```python
from build123d import *

# Parameters (mm, degrees)
SKETCH1_W                                      = 152.4
SKETCH1_H                                      = 152.4
BOSS_EXTRUDE1_DEPTH                            = 12.7
F_2_56_TAPPED_HOLE1_D                          = 1.778
CBORE_FOR_4_SOCKET_HEAD_CAP_SCREW1_D           = 3.2639
CBORE_FOR_4_SOCKET_HEAD_CAP_SCREW1_CBORE_D     = 5.55752
CBORE_FOR_4_SOCKET_HEAD_CAP_SCREW1_CBORE_DEPTH = 2.8448
F_6_0MM_DOWEL_HOLE1_D                          = 6
F_8_0MM_DOWEL_HOLE1_D                          = 8
F_1_4_20_TAPPED_HOLE1_D                        = 5.1054


with BuildPart() as part:
    # Sketch1 → Boss-Extrude1 (new body)
    with BuildSketch(Plane.XY):
        Rectangle(SKETCH1_W, SKETCH1_H)
    extrude(amount=BOSS_EXTRUDE1_DEPTH)

    # #2-56 Tapped Hole1 (through all)
    with Locations(Plane.XY.offset(12.7)):
        with Locations((-50.8, 0), (-50.8, -58), (-1.8, -58), (-1.8, 0)):
            Hole(F_2_56_TAPPED_HOLE1_D / 2)

    # CBORE for #4 Socket Head Cap Screw1 (through all)
    with Locations(Plane.XY.offset(12.7)):
        with Locations((-73.025, 63.5), (-73.025, 73.025), (73.025, 63.5), (73.025, 73.025), (73.025, -63.5), (73.025, -73.025), (-73.025, -63.5), (-73.025, -73.025)):
            CounterBoreHole(CBORE_FOR_4_SOCKET_HEAD_CAP_SCREW1_D / 2, CBORE_FOR_4_SOCKET_HEAD_CAP_SCREW1_CBORE_D / 2, CBORE_FOR_4_SOCKET_HEAD_CAP_SCREW1_CBORE_DEPTH)

    # Ø6.0mm Dowel Hole1 (through all)
    with Locations(Plane.XY.offset(12.7)):
        with Locations((57.15, 63.5), (57.15, -24.801), (-19.32090918, 19.3495), (57.15, -57.15), (25.4, -57.15)):
            Hole(F_6_0MM_DOWEL_HOLE1_D / 2)

    # Ø8.0mm Dowel Hole1 (through all)
    with Locations(Plane.XY.offset(12.7)):
        with Locations((31.65969694, 19.3495)):
            Hole(F_8_0MM_DOWEL_HOLE1_D / 2)

    # 1/4-20 Tapped Hole1 (through all)
    with Locations(Plane.XY.offset(12.7)):
        with Locations((31.65969694, 0.2995), (31.65969694, 38.3995)):
            Hole(F_1_4_20_TAPPED_HOLE1_D / 2)


solid = part.part
```
CAD build for the part. Positions are in the model's coordinates, mm. A direction names the side the tool comes from. Give positions to 0.01 mm unless a question says otherwise; leave off trailing zeros. Order: outer loops, then holes, each group sorted by start corner. A loop starts at its lowest first (then second) coordinate and runs counter-clockwise, first axis right, second up.
(1) Saw through at A-A, the plane x = 57.15. Give the cut face in (y, z).
(2) Tool access for faces 1 (the cylindrical face through (-75.8, 73.15, 11.3)), 2 (the cylindrical face through (27.844, 20.551, 6.261)): list every direction of +Z, -Z, +X, -X, +Y, -Y with a clear straight run to the whole face (end or side of a thin tool).
(3) Flat gauge pins, fed straight in: pin 1 (4.5 mm diameter, centred on x = 73.5, y = 64.5, fed in from +Z); pin 2 (5 mm diameter, centred on x = 73.025, y = -73.025, fed in from +Z). Where does each tip first touch, or does it go through?
(4) Saw through at B-B, the plane x = -19. Give the cut face in (y, z), then the cut area to 3 significant figures.
(5) Drill centre lines: L1, parallel to X at y = 37.5, z = 2.5; L2, parallel to X at y = 23, z = 10.25. Where is each one in solid material? Low to high.
(6) Mould opens along X. For faces 3 (the flat face through (-1, -76.2, 6)), 4 (the cylindrical face through (-16.324, 19.481, 6.261)), 5 (the flat face through (76.2, -1, 6)), 6 (the cylindrical face through (73.237, -71.407, 4.859)) say: released by +X, released by -X, zero draft, split by the parting line, or undercut.
Results found:
1. outline: (-76.2, 0) - (-60.15, 0) - (-60.15, 12.7) - (-76.2, 12.7) - close; (-54.15, 0) - (-27.8, 0) - (-27.8, 12.7) - (-54.15, 12.7) - close; (-21.8, 0) - (60.5, 0) - (60.5, 12.7) - (-21.8, 12.7) - close; (66.5, 0) - (76.2, 0) - (76.2, 12.7) - (66.5, 12.7) - close
2. face 1: +Z
2. face 2: +Z, -Z
3. pin 1: stops at z = 12.7
3. pin 2: stops at z = 9.86
4. outline: (-76.2, 0) - (16.37, 0) - (16.37, 12.7) - (-76.2, 12.7) - close; (22.33, 0) - (76.2, 0) - (76.2, 12.7) - (22.33, 12.7) - close
4. area: 1,860 mm2
5. L1: x = -76.2 to 29.27, 34.05 to 76.2
5. L2: x = -76.2 to 30.02, 33.29 to 76.2
6. face 3: zero draft
6. face 4: undercut
6. face 5: released by +X
6. face 6: undercut
